Job drawing, mm, ordinate dimensions from the low corner. One solid piece. A direction names the side the tool comes from. Give positions to 0.01 mm unless a question says otherwise; leave off trailing zeros. Order: outer loops, then holes, each group sorted by start corner. A loop starts at its lowest first (then second) coordinate and runs counter-clockwise, first axis right, second up.
1. Which spindle directions (+Z, -Z, +X, -X, +Y, -Y) get a long thin tool onto all of the face, cutting with end or side? Do the marked faces 3 and 4. Say none if no direction does.
2. Probe line 1 (X direction, y = 68, z = 5.75) (1 decimal); line 2 (Y direction, x = 79.5, z = 4.75) (1 decimal); line 3 (Y direction, x = 23, z = 5) (1 decimal). List the from-to ranges inside material, lowest first.
3. Drop flat-ended pins along their axis: pin 1 Ø3 at (y, z) = (64.5, 1.5) entering from +X (1 decimal); pin 2 Ø1.9 at (x, z) = (57, 3) entering from +Y (1 decimal). Give the stop position or say it passes through.
4. Slice it at B-B on x = 22. Give the number of separate pieces and of enclosed holes in the cut face.
5. Mould opens along X. For the marked faces 1 and 2 say: +X half, -X half, draft (parallel to the pull), parting line (faces both ways), or undercut.
6. Slice it at D-D on z = 1.25. List the corners of the cut face in (x, y) (1 decimal).
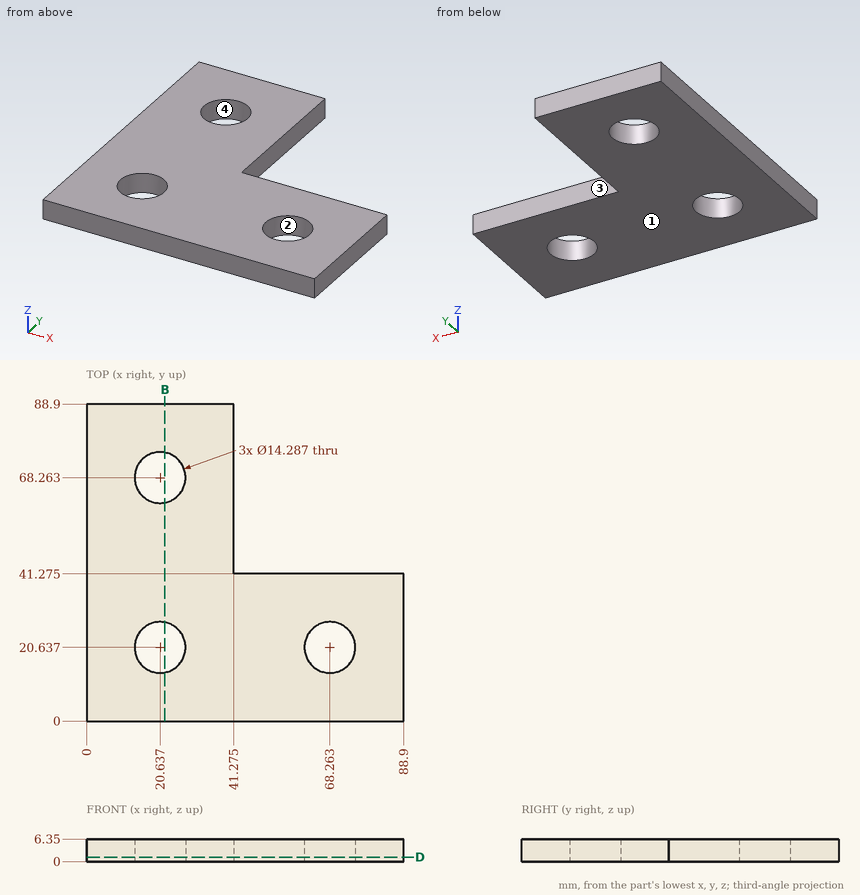
Data:
1. face 3: +Z, -Z, +X, +Y
1. face 4: +Z, -Z
2. line 1: x = 0 to 13.5, 27.8 to 41.3
2. line 2: y = 0 to 41.3
2. line 3: y = 0 to 13.9, 27.4 to 61.5, 75 to 88.9
3. pin 1: stops at x = 41.3
3. pin 2: stops at y = 41.3
4. separate pieces: 3
4. enclosed holes: 0
5. face 1: draft
5. face 2: undercut
6. outline: (0, 0) - (88.9, 0) - (88.9, 41.3) - (41.3, 41.3) - (41.3, 88.9) - (0, 88.9) - close; hole circle Ø14.3 at (20.6, 20.6); hole circle Ø14.3 at (20.6, 68.3); hole circle Ø14.3 at (68.3, 20.6)
